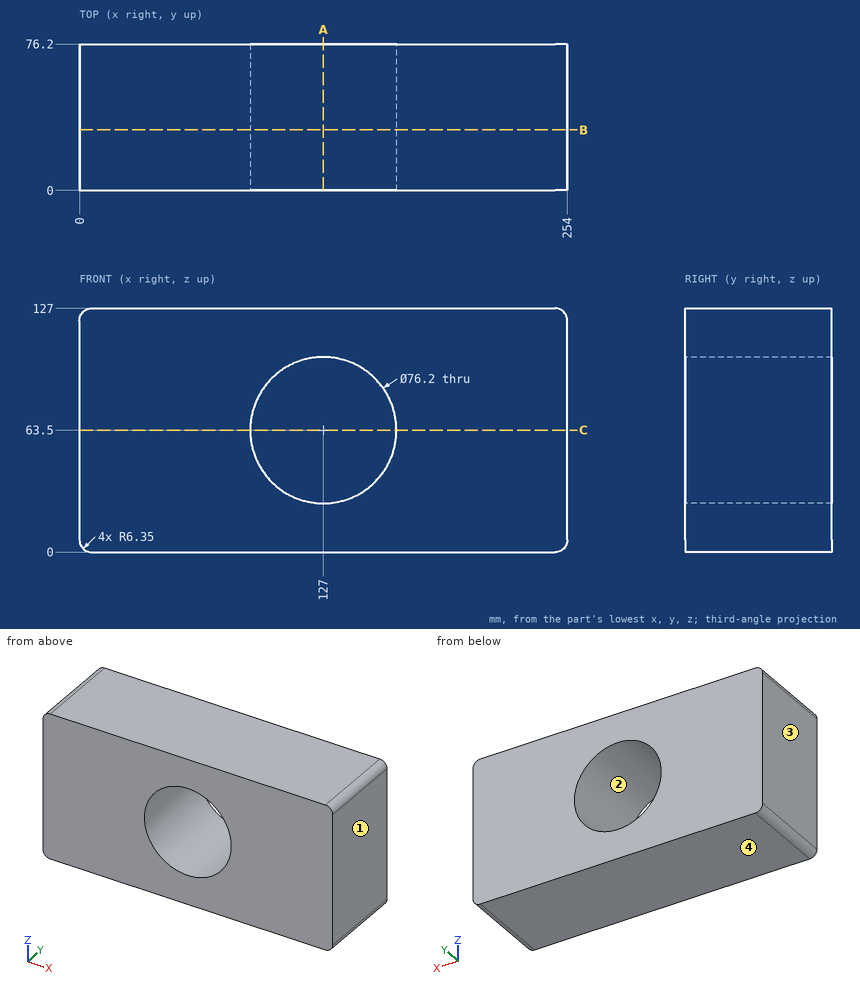
Design review of the part shown in the three views and the two pictorial views. Dimensions are in mm from the part's minimum x, y and z. Coordinates: 2 decimals unless noted, no trailing zeros. Loops run counter-clockwise (first coordinate to the right, second up) from the corner with the lowest first, then second, coordinate; pieces in that order, holes last. Notation, with made-up numbers: (61, 27.25) - (82, 27.25) arc R33 cw to (82, 60.25) - close; hole circle Ø8 at (65, 32.25). An arc over 180 degrees is marked (long way). Use a Markdown table: item, result. Add a question column.
Item 1: For line 1 (Z direction, x = 127, y = 29); line 2 (X direction, y = 33, z = 63); line 3 (X direction, y = 18, z = 98), list the stretches that pass through material, from the lowest coordinate up.
Item 2: We need section C-C (z = 63.5). Give the boundary of the cut face in (x, y).
Item 3: We need section B-B (y = 31.5). Give the boundary of the cut face in (x, z), and give its area (3 significant figures).
Item 4: Mouldability with a two-part tool opening along X and no side actions: class the marked faces 1, 2, 3 and 4 as pulls with the +X half, pulls with the -X half, needs draft (parallel to the pull), parting line crosses it, or undercut.
Item 5: We need section A-A (x = 127). Give the boundary of the cut face in (y, z).
Results list:
| question | item | result |
|---|---|---|
| 1 | line 1 | z = 0 to 25.4, 101.6 to 127 |
| 1 | line 2 | x = 0 to 88.9, 165.1 to 254 |
| 1 | line 3 | x = 0 to 110.83, 143.17 to 254 |
| 2 | outline | (0, 0) - (88.9, 0) - (88.9, 76.2) - (0, 76.2) - close; (165.1, 0) - (254, 0) - (254, 76.2) - (165.1, 76.2) - close |
| 3 | outline | (0, 6.35) arc R6.35 ccw to (6.35, 0) - (247.65, 0) arc R6.35 ccw to (254, 6.35) - (254, 120.65) arc R6.35 ccw to (247.65, 127) - (6.35, 127) arc R6.35 ccw to (0, 120.65) - close; hole circle Ø76.2 at (127, 63.5) |
| 3 | area | 27,700 mm^2 |
| 4 | face 1 | pulls with the +X half |
| 4 | face 2 | undercut |
| 4 | face 3 | pulls with the -X half |
| 4 | face 4 | needs draft |
| 5 | outline | (0, 0) - (76.2, 0) - (76.2, 25.4) - (0, 25.4) - close; (0, 101.6) - (76.2, 101.6) - (76.2, 127) - (0, 127) - close |
